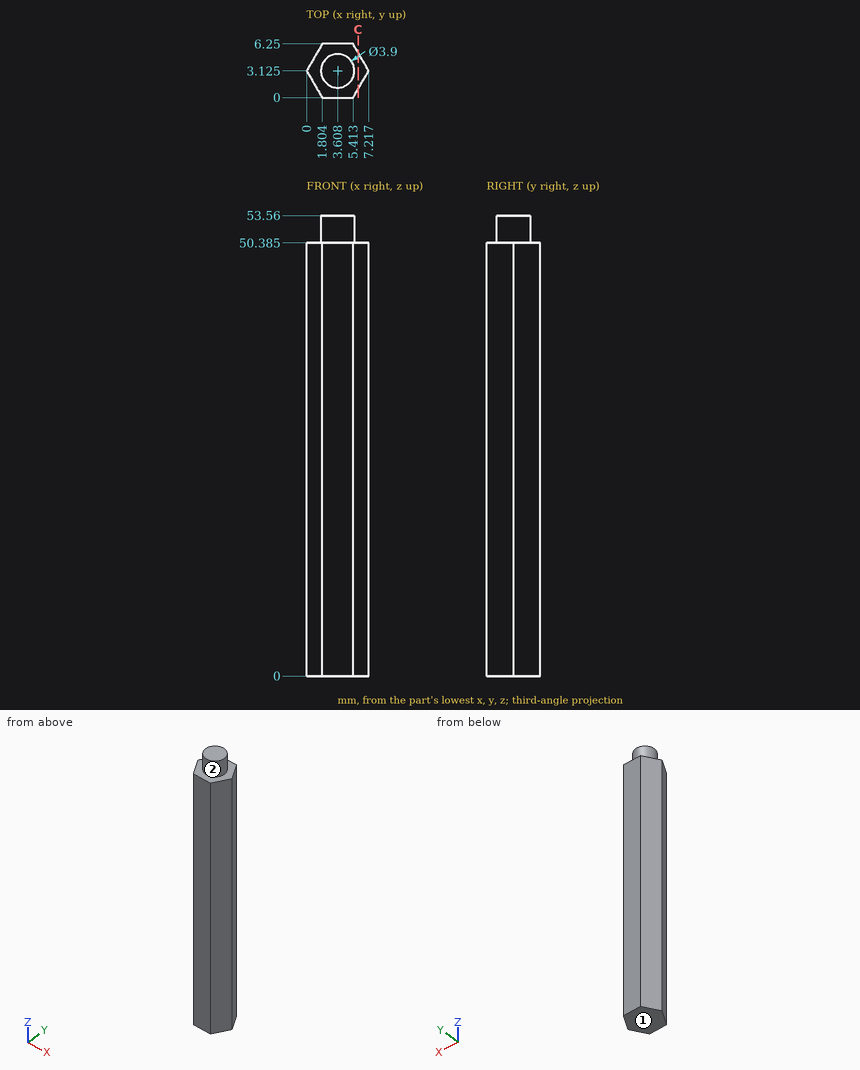
Verification items for this drawing (mm, ordinates from the low corner). A direction names the side the tool comes from. Round coordinates to 2 decimals unless told otherwise and drop trailing zeros. Order: outer loops, then holes, each group sorted by start corner. A loop starts at its lowest first (then second) coordinate and runs counter-clockwise, first axis right, second up.
1) Cross-section at C-C, the plane x = 6. Record the cut outline in (y, z) (1 decimal), plus the area to 3 significant figures.
Geometry says:
outline: (1, 0) - (5.2, 0) - (5.2, 50.4) - (1, 50.4) - close
area: 212 mm2
2) Material ranges on line 1 (Z direction, x = 4, y = 0.5) (1 decimal); line 2 (X direction, y = 5.25, z = 31.5) (1 decimal); line 3 (Y direction, x = 5.75, z = 36) (1 decimal), recorded low to high.
Geometry says:
line 1: z = 0 to 50.4
line 2: x = 1.2 to 6
line 3: y = 0.6 to 5.7
3) Tool access check on the marked faces 1 and 2. Record the directions out of +Z, -Z, +X, -X, +Y, -Y that give a thin tool (end or side, any length) a straight path to the whole face; none if there is none.
Geometry says:
face 1: -Z, +X, -X, +Y, -Y
face 2: +Z
4) Depth check by flat-ended pin: pin 1 (1.5 mm diameter, centred on x = 2.5, y = 5, fed in from -Z); pin 2 (1 mm diameter, centred on y = 5, z = 34.5, fed in from +X); pin 3 (2 mm diameter, centred on y = 1.5, z = 40.5, fed in from +X) (1 decimal). Enter the tip coordinate at first touch or a pass-through.
Geometry says:
pin 1: stops at z = 0
pin 2: stops at x = 6.42
pin 3: stops at x = 6.9
